Could you check a few things on this drawing? It's one solid part, dimensions in mm from its lowest x, y, z. A direction names the side the tool comes from. Coordinates: 2 decimals unless noted, no trailing zeros. Order: outer loops, then holes, each group sorted by start corner. A loop starts at its lowest first (then second) coordinate and runs counter-clockwise, first axis right, second up. Notation, with made-up numbers: (55.5, -3) - (93.5, -3) arc R22 cw to (93.5, 22) - close; hole circle Ø1 at (23.5, 68.25). An arc over 180 degrees is marked (long way). Return JSON: item names as keys, results as strings. Group by question number.
1) Which directions (+Z, -Z, +X, -X, +Y, -Y) give clear straight access to the entire face, cutting with the end or side of a thin tool? Please do the marked faces 1 and 2.
2) Imagine slicing it at B-B (x = 21.5). Write out the boundary of the cut face in (y, z).
3) For pin 1 Ø6 at (y, z) = (6.5, 48) entering from -X; pin 2 Ø4 at (x, z) = (20, 65) entering from +Y, each with a flat end and sliding along its axis, tell me the tip position at first contact or that it passes through.
4) Imagine slicing it at C-C (z = 61.5). Write out the boundary of the cut face in (x, y).
5) If I drill on line 1 along Z through (x, y) = (20.5, 9); line 2 along X through (y, z) = (6, 27); line 3 along Z through (x, y) = (15.5, 6.5) (1 decimal), over which ranges is the centre line in solid material (lowest first)?
6) Imagine slicing it at A-A (y = 7). Give the number of separate pieces and of enclosed holes in the cut face, and give its area (3 significant figures).
7) If we mould it in two halves opening along Z, with no side actions, what happens to the marked faces 3, 4, 5 and 6? For each: pulls with the +Z half, pulls with the -Z half, needs draft (parallel to the pull), parting line crosses it, or undercut.
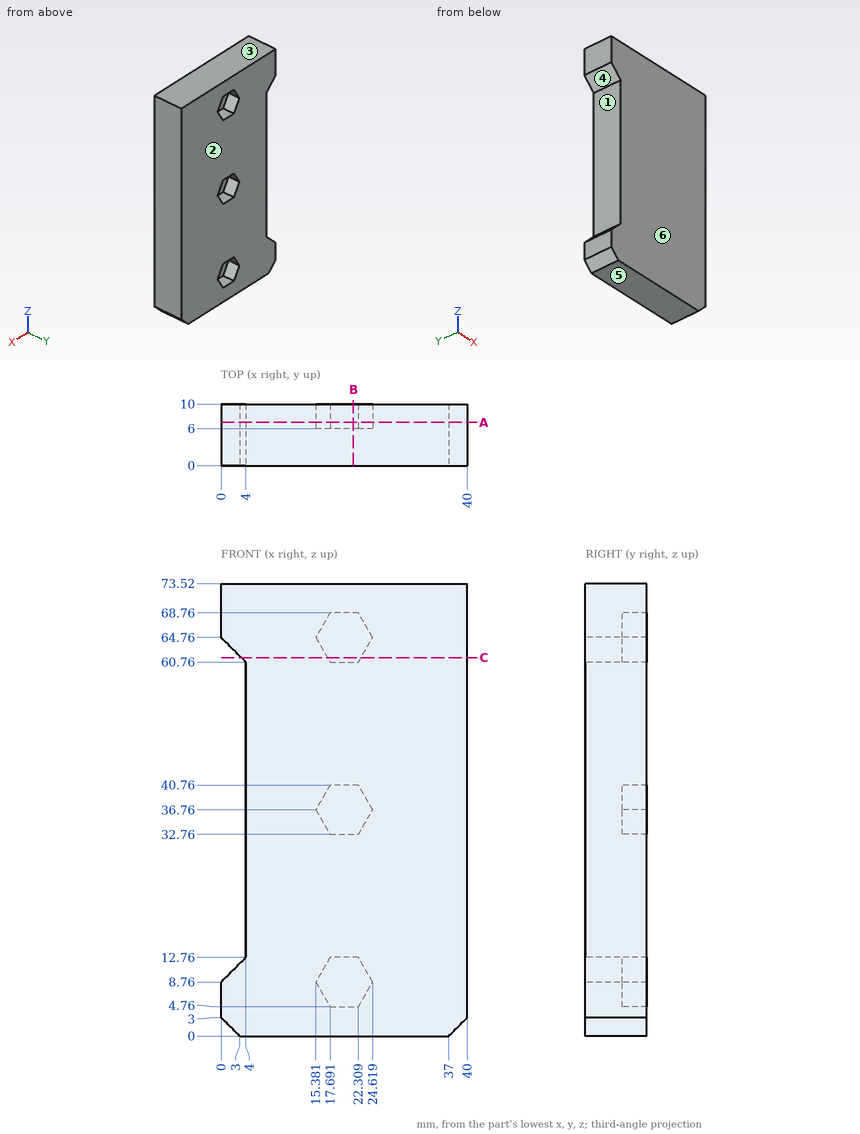
Calculated:
{
 "1": {"face 1": "-X, +Y, -Y", "face 2": "+Z, -Z, +X, -X, +Y"},
 "2": {"outline": "(0, 0) - (10, 0) - (10, 4.76) - (6, 4.76) - (6, 12.76) - (10, 12.76) - (10, 32.76) - (6, 32.76) - (6, 40.76) - (10, 40.76) - (10, 60.76) - (6, 60.76) - (6, 68.76) - (10, 68.76) - (10, 73.52) - (0, 73.52) - close"},
 "3": {"pin 1": "x = 4", "pin 2": "y = 6"},
 "4": {"outline": "(3.26, 0) - (40, 0) - (40, 10) - (22.74, 10) - (22.74, 6) - (17.26, 6) - (17.26, 10) - (3.26, 10) - close"},
 "5": {"line 1": "0 to 4.76, 12.76 to 32.76, 40.76 to 60.76, 68.76 to 73.52", "line 2": "4 to 40", "line 3": "0 to 8.6, 9 to 36.6, 37 to 64.6, 65 to 73.5"},
 "6": {"separate pieces": "1", "enclosed holes": "3", "area": "2,560 mm2"},
 "7": {"face 3": "pulls with the +Z half", "face 4": "undercut", "face 5": "pulls with the -Z half", "face 6": "needs draft"}
}
